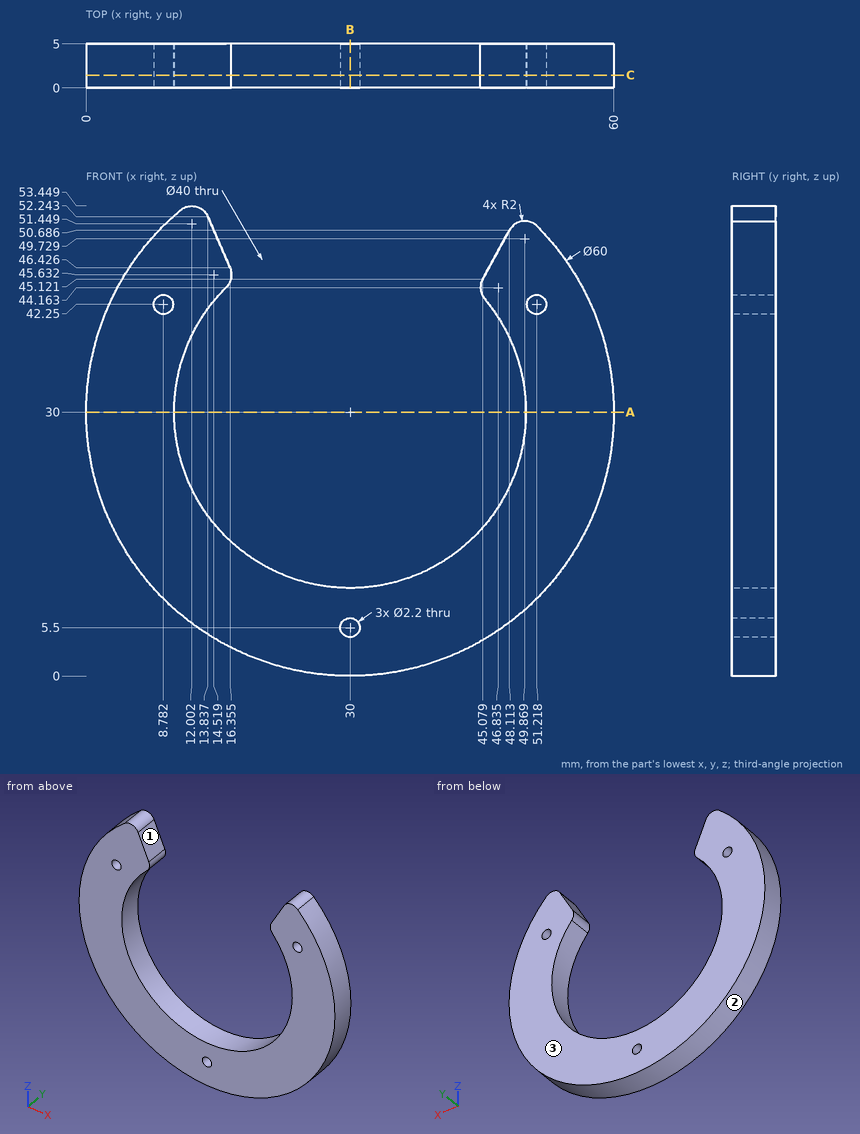
Study the drawing (mm; zero at the part's minimum x, y, z) and answer. Give positions to 0.01 mm unless a question says otherwise; leave off trailing zeros. Write each loop counter-clockwise with the first axis right and the second up, starting at its lowest first coordinate (ties: lowest second). Pieces come first, ordered by that corner, then holes. Notation, with made-up numbers: M -36.75,50 L -10.75,50 A20 ccw -10.75,67 Z; hole C -35.5,59 d7. An arc over 180 degrees is marked long. Put each result on its own line as item: value. Start each with the question number.
1. The part is cut by section A-A, the plane z = 30. Give the vertices of the cut face in (x, y).
2. The part is cut by section C-C, the plane y = 1.45. Give the number of separate pieces and of enclosed holes in the cut face, and give its area (3 significant figures).
3. Consider line 1 along X through (y, z) = (3.45, 42.25) (1 decimal); line 2 along X through (y, z) = (4.5, 20) (1 decimal); line 3 along X through (y, z) = (3.9, 32.5) (1 decimal). Determine where each line is inside the solid, lowest interval first.
4. The part is cut by section B-B, the plane x = 30. Give the vertices of the cut face in (y, z).
5. For a pull along X with two mould halves and no side action, classify the marked faces 1, 2 and 3 as released by +X, released by -X, zero draft, split by the parting line, or undercut.
6. Each of these flat-tipped pins is pushed along its axis until it touches: pin 1 Ø3 at (y, z) = (2, 10) entering from -X; pin 2 Ø6 at (x, z) = (41.5, 42.5) entering from -Y; pin 3 Ø1 at (y, z) = (3, 44) entering from +X. Where does it stop, or does it pass through?
Final values:
1. outline: M 0,0 L 10,0 L 10,5 L 0,5 Z; M 50,0 L 60,0 L 60,5 L 50,5 Z
2. separate pieces: 1
2. enclosed holes: 3
2. area: 1,210 mm²
3. line 1: x = 2.6 to 7.7, 9.9 to 14.2, 45.8 to 50.1, 52.3 to 57.4
3. line 2: x = 1.7 to 12.7, 47.3 to 58.3
3. line 3: x = 0.1 to 10.2, 49.8 to 59.9
4. outline: M 0,0 L 5,0 L 5,4.4 L 0,4.4 Z; M 0,6.6 L 5,6.6 L 5,10 L 0,10 Z
5. face 1: undercut
5. face 2: split by the parting line
5. face 3: zero draft
6. pin 1: stops at x = 6.38
6. pin 2: passes through
6. pin 3: stops at x = 56.79
